Part model, mm, in its own coordinate system. A direction names the side the tool comes from. Round coordinates to 2 decimals unless told otherwise and drop trailing zeros. Write each loop counter-clockwise with the first axis right and the second up, starting at its lowest first coordinate (ties: lowest second). Pieces come first, ordered by that corner, then holes.
```python
from build123d import *

# Parameters (mm, degrees)
SKETCH1_W           = 6.35
SKETCH1_H           = 9.525
BOSS_EXTRUDE1_DEPTH = 1.5748
SKETCH2_R           = 1.1303
CUT_EXTRUDE1_DEPTH  = 2.5748
SKETCH3_W           = 6.35
SKETCH3_H           = 1.5748
BOSS_EXTRUDE2_DEPTH = 7.1374
SKETCH4_R           = 1.1303
CUT_EXTRUDE2_DEPTH  = 2.5748


with BuildPart() as part:
    # Sketch1 → Boss-Extrude1 (new body)
    with BuildSketch(Plane(origin=(0, 0, 0), x_dir=(1, 0, 0), z_dir=(0, 1, 0))):
        Rectangle(SKETCH1_W, SKETCH1_H)
    extrude(amount=BOSS_EXTRUDE1_DEPTH)

    # Sketch2 → Cut-Extrude1 (cut, through all)
    with BuildSketch(Plane(origin=(0, 1.5748, 0), x_dir=(1, 0, 0), z_dir=(0, 1, 0))):
        with Locations((0, -1.5875)):
            Circle(SKETCH2_R)
    extrude(amount=-CUT_EXTRUDE1_DEPTH, mode=Mode.SUBTRACT)

    # Sketch3 → Boss-Extrude2 (add)
    with BuildSketch(Plane(origin=(0, 1.5748, 0), x_dir=(1, 0, 0), z_dir=(0, 1, 0))):
        with Locations((0, 3.9751)):
            Rectangle(SKETCH3_W, SKETCH3_H)
    extrude(amount=BOSS_EXTRUDE2_DEPTH)

    # Sketch4 → Cut-Extrude2 (cut, through all)
    with BuildSketch(Plane.XY.offset(-3.1877)):
        with Locations((0, 5.1562)):
            Circle(SKETCH4_R)
    extrude(amount=-CUT_EXTRUDE2_DEPTH, mode=Mode.SUBTRACT)


solid = part.part
```
Q1. Mould opens along Z. For faces 3 (the flat face through (-1, 4, -4.762)), 4 (the flat face through (-3.175, 1, -1)), 5 (the cylindrical face through (-0.2, 0.8, 2.7)) say: +Z half, -Z half, draft (parallel to the pull), parting line (faces both ways), or undercut.
Values follow:
face 3: -Z half
face 4: draft
face 5: undercut
Q2. Cut at B-B on y = 5. Write the cut outline in (x, z) (1 decimal).
Values follow:
outline: (-3.2, -4.8) - (-1.1, -4.8) - (-1.1, -3.2) - (-3.2, -3.2) - close; (1.1, -4.8) - (3.2, -4.8) - (3.2, -3.2) - (1.1, -3.2) - close
Q3. Which spindle directions (+Z, -Z, +X, -X, +Y, -Y) get a long thin tool onto all of the face, cutting with end or side? Do faces 1 (the flat face through (0, 0, 0)), 2 (the flat face through (0, 1.575, 0)). Say none if no direction does.
Values follow:
face 1: +Z, -Z, +X, -X, -Y
face 2: +Z, +X, -X, +Y
Q4. Wall check: L1, parallel to Z at x = 0, y = 0.5; L2, parallel to Y at x = 0, z = -4.2; L3, parallel to Y at x = 2, z = -2.75. Give the ranges that are in metal, low to high.
Values follow:
L1: z = -4.76 to 0.46, 2.72 to 4.76
L2: y = 0 to 4.03, 6.29 to 8.71
L3: y = 0 to 1.57
Q5. Drop flat-ended pins along their axis: pin 1 (2 mm diameter, centred on x = 0, y = 5.16, fed in from -Z); pin 2 (1.9 mm diameter, centred on x = 0.5, z = 2.5, fed in from +Y). Give the stop position or say it passes through.
Values follow:
pin 1: passes through
pin 2: stops at y = 1.57
Q6. Cut at D-D on x = -1.5. Write the cut outline in (y, z), plus the area to 3 significant figures.
Values follow:
outline: (0, -4.76) - (8.71, -4.76) - (8.71, -3.19) - (1.57, -3.19) - (1.57, 4.76) - (0, 4.76) - close
area: 26.2 mm2
Q7. Cut at C-C on z = -1. Write the cut outline in (x, y) (3 decimals), plus the area to 4 significant figures.
Values follow:
outline: (-3.175, 0) - (3.175, 0) - (3.175, 1.575) - (-3.175, 1.575) - close
area: 10.00 mm2
Q8. Cut at A-A on x = 0. Write the cut outline in (y, z), plus the area to 3 significant figures.
Values follow:
outline: (0, -4.76) - (4.03, -4.76) - (4.03, -3.19) - (1.57, -3.19) - (1.57, 0.46) - (0, 0.46) - close; (0, 2.72) - (1.57, 2.72) - (1.57, 4.76) - (0, 4.76) - close; (6.29, -4.76) - (8.71, -4.76) - (8.71, -3.19) - (6.29, -3.19) - close
area: 19.1 mm2
